Could you check a few things on this model? Use its own coordinates, in mm. A direction names the side the tool comes from. Round coordinates to 2 decimals unless told otherwise and drop trailing zeros. Loops run counter-clockwise (first coordinate to the right, second up) from the corner with the lowest first, then second, coordinate; pieces in that order, holes last. Notation, with made-up numbers: (20, -18) - (26, -18) arc R24 cw to (26, 9) - close; hole circle Ø11 at (71.25, 80). An arc over 180 degrees is marked (long way). Put each result on its own line as item: value. Start each with the question number.
from build123d import *

# Parameters (mm, degrees)
SKETCH1_R           = 0.5
BOSS_EXTRUDE1_DEPTH = 3
SKETCH2_W           = 20
SKETCH2_H           = 3
BOSS_EXTRUDE2_DEPTH = 5


with BuildPart() as part:
    # Sketch1 → Boss-Extrude1 (new body)
    with BuildSketch(Plane.XY):
        with BuildLine():
            Line((0.468871097, 6.999999884), (-5.5, 6.999999884))
            Line((-5.5, 6.999999884), (-5.5, 3))
            Line((-5.5, 3), (0, 3))
            Line((0, 3), (0, 0))
            Line((0, 0), (9, 0))
            Line((9, 0), (9, 3))
            Line((9, 3), (14.5, 3))
            Line((14.5, 3), (14.5, 6.999999884))
            Line((14.5, 6.999999884), (8.531128903, 6.999999884))
            ThreePointArc((8.531128903, 6.999999884), (4.5, 9.499999942), (0.468871097, 6.999999884))
        make_face()
        with Locations((4.5, 4.999999942)):
            Circle(SKETCH1_R, mode=Mode.SUBTRACT)
    extrude(amount=BOSS_EXTRUDE1_DEPTH)

    # Sketch2 → Boss-Extrude2 (add)
    with BuildSketch(Plane.XZ):
        with Locations((4.5, 1.5)):
            Rectangle(SKETCH2_W, SKETCH2_H)
    extrude(amount=BOSS_EXTRUDE2_DEPTH)


solid = part.part
Item 1: Suppose I cut it at A-A, the plane x = -3. List the corners of the cut face in (y, z) for me.
Item 2: Suppose I cut it at C-C, the plane z = 0.3. List the corners of the cut face in (x, y) for me.
Item 3: Suppose I cut it at B-B, the plane y = 5. List the corners of the cut face in (x, z) for me, then the cut area to 3 significant figures.
Item 4: Will these pins go through, and if not, where does the flat tip stop? P1, Ø0.9, axis at y = 1, z = 1.5, coming from the -X side; P2, Ø0.9, axis at x = -4, z = 1, coming from the +Y side; P3, Ø1.5, axis at y = 1.5, z = 1.5, coming from the +X side.
Item 5: On a 3-axis mill with a long thin cutter (end or side, diameter ignored), from which of +Z, -Z, +X, -X, +Y, -Y can I reach the whole of each face in a straight line? I mean faces 4 (the face through (12, 0, 2)), 5 (the face through (-2, 7, 1)), 6 (the face through (12, 7, 1)). Say none if no direction works.
Item 6: I need wall thicknesses on line 1 (Y direction, x = 4.5, z = 1); line 2 (Y direction, x = 13.5, z = 2.85); line 3 (X direction, y = 5, z = 0.85). Which ranges of each line are inside material? Lowest first, please. Write a range as from..to.
Item 7: Suppose I cut it at D-D, the plane y = 1.75. List the corners of the cut face in (x, z) for me.
Item 8: Thinking about a two-plate mould opening in Y: for faces 1 (the face through (4.6, 9.5, 1.5)), 2 (the face through (-3, 3, 1)), 3 (the face through (4, 1, 3)), which applies, released by +Y, released by -Y, zero draft, split by the parting line, or undercut?
Numbers:
1. outline: (-5, 0) - (0, 0) - (0, 3) - (-5, 3) - close; (3, 0) - (7, 0) - (7, 3) - (3, 3) - close
2. outline: (-5.5, -5) - (14.5, -5) - (14.5, 0) - (9, 0) - (9, 3) - (14.5, 3) - (14.5, 7) - (8.53, 7) arc R4.5 ccw to (0.47, 7) - (-5.5, 7) - (-5.5, 3) - (0, 3) - (0, 0) - (-5.5, 0) - close; hole circle Ø1 at (4.5, 5)
3. outline: (-5.5, 0) - (4, 0) - (4, 3) - (-5.5, 3) - close; (5, 0) - (14.5, 0) - (14.5, 3) - (5, 3) - close
3. area: 57.0 mm^2
4. P1: x = 0
4. P2: y = 7
4. P3: x = 9
5. face 4: +Z, -Z, +X
5. face 5: +Z, -Z, -X, +Y
5. face 6: +Z, -Z, +X, +Y
6. line 1: -5..4.5, 5.5..9.5
6. line 2: -5..0, 3..7
6. line 3: -5.5..4, 5..14.5
7. outline: (0, 0) - (9, 0) - (9, 3) - (0, 3) - close
8. face 1: released by +Y
8. face 2: undercut
8. face 3: zero draft
